Could you check a few things on this drawing? It's one solid part, dimensions in mm from its lowest x, y, z. A direction names the side the tool comes from. Round coordinates to 2 decimals unless told otherwise and drop trailing zeros. Write each loop counter-clockwise with the first axis right and the second up, starting at its lowest first coordinate (ties: lowest second). Pieces come first, ordered by that corner, then holes. Notation, with made-up numbers: (0, 61) -> (58, 61) arc R24 ccw to (58, 93) -> close; hole circle Ø10 at (84.5, 65.5). An arc over 180 degrees is marked (long way). Answer as CSV lines item,"result".
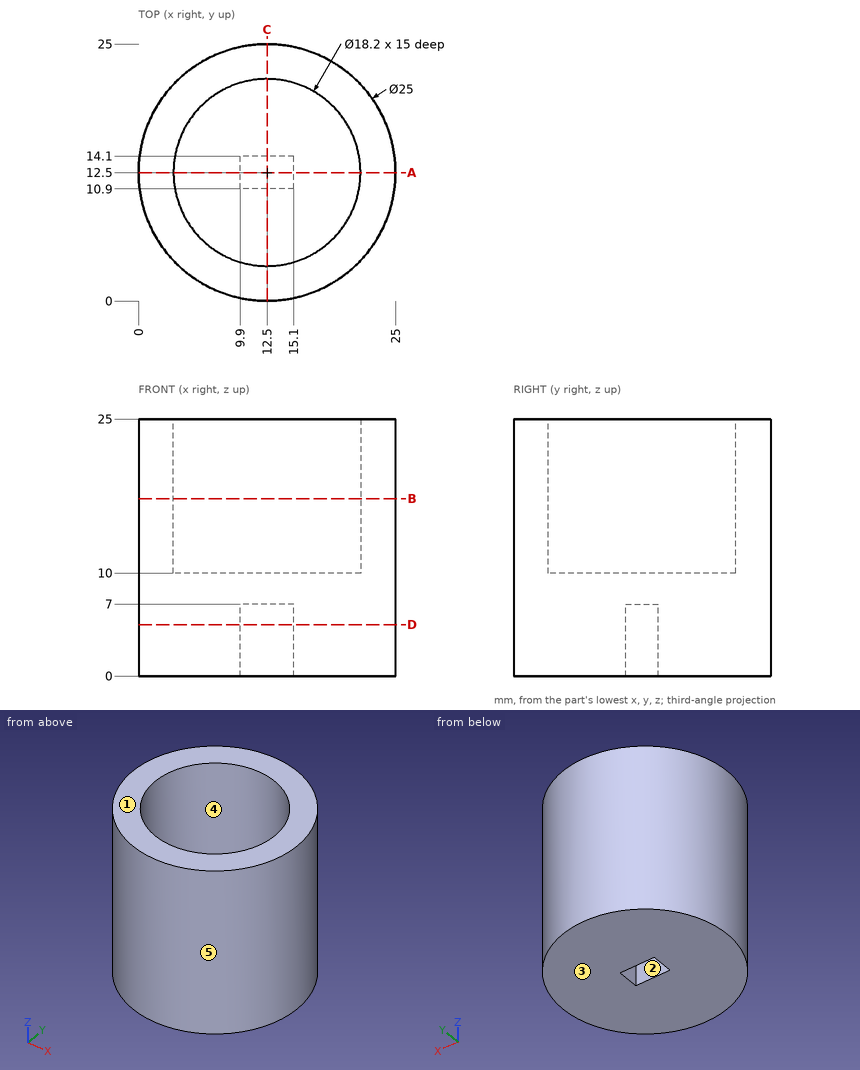
1. If I drill on line 1 (Y direction, x = 12.5, z = 22); line 2 (Y direction, x = 16, z = 10.25); line 3 (Z direction, x = 10.5, y = 14.75), over which ranges is the centre line in solid material (lowest first)?
Numbers:
line 1,"y = 0 to 3.4, 21.6 to 25"
line 2,"y = 0.5 to 4.1, 20.9 to 24.5"
line 3,"z = 0 to 10"
2. On a 3-axis mill with a long thin cutter (end or side, diameter ignored), from which of +Z, -Z, +X, -X, +Y, -Y can I reach the whole of each face in a straight line? I mean the marked faces 1 and 2. Say none if no direction works.
Numbers:
face 1,"+Z, +X, -X, +Y, -Y"
face 2,"-Z"
3. Suppose I cut it at D-D on z = 5. Please give me the cut outline in (x, y), and give its area (3 significant figures).
Numbers:
outline,"circle Ø25 at (12.5, 12.5); hole (9.9, 10.9) -> (15.1, 10.9) -> (15.1, 14.1) -> (9.9, 14.1) -> close"
area,"474 mm^2"
4. If we mould it in two halves opening along X, with no side actions, what happens to the marked faces 3, 4 and 5? For each: released by +X, released by -X, zero draft, split by the parting line, or undercut.
Numbers:
face 3,"zero draft"
face 4,"undercut"
face 5,"split by the parting line"
5. For pin 1 Ø6 at (y, z) = (16, 19) entering from -X; pin 2 Ø3 at (y, z) = (3, 14.5) entering from -X; pin 3 Ø1 at (y, z) = (13.5, 4) entering from +X, each with a flat end and sliding along its axis, tell me the tip position at first contact or that it passes through.
Numbers:
pin 1,"stops at x = 0.01"
pin 2,"stops at x = 2.9"
pin 3,"stops at x = 24.99"
6. Suppose I cut it at C-C on x = 12.5. Please give me the cut outline in (y, z), and give its area (3 significant figures).
Numbers:
outline,"(0, 0) -> (10.9, 0) -> (10.9, 7) -> (14.1, 7) -> (14.1, 0) -> (25, 0) -> (25, 25) -> (21.6, 25) -> (21.6, 10) -> (3.4, 10) -> (3.4, 25) -> (0, 25) -> close"
area,"330 mm^2"
7. Suppose I cut it at B-B on z = 17.25. Please give me the cut outline in (x, y), and give its area (3 significant figures).
Numbers:
outline,"circle Ø25 at (12.5, 12.5); hole circle Ø18.2 at (12.5, 12.5)"
area,"231 mm^2"
8. Suppose I cut it at A-A on y = 12.5. Please give me the cut outline in (x, z).
Numbers:
outline,"(0, 0) -> (9.9, 0) -> (9.9, 7) -> (15.1, 7) -> (15.1, 0) -> (25, 0) -> (25, 25) -> (21.6, 25) -> (21.6, 10) -> (3.4, 10) -> (3.4, 25) -> (0, 25) -> close"
